Input: part model. Units: mm. Frame: model coordinates. Face numbers are marked on the shaded views. A direction names the side the tool comes from. Give positions to 0.01 mm unless a question says otherwise; leave off trailing zeros. Loops run counter-clockwise (first coordinate to the right, second up) from the corner with the lowest first, then second, coordinate; pieces in that order, holes last. Notation, with made-up numbers: (-18, 72) -> (-6, 72) arc R18 cw to (-6, 90) -> close; hole circle Ø10 at (38, 1). An arc over 180 degrees is marked (long way). Answer as a JSON object with one key per item and string values. Group by question number.
Autodesk Inventor part; units mm, degrees
ref_plane "YZ Plane" through (0, 0, 0) normal (1, 0, 0) x (0, 1, 0)
ref_plane "XZ Plane" through (0, 0, 0) normal (0, 1, 0) x (-1, 0, 0)
ref_plane "XY Plane" through (0, 0, 0) normal (0, 0, 1) x (1, 0, 0)
sketch "Sketch1" plane through (0, 0, 0) normal (0, 0, 1) x (1, 0, 0)
  line L0 (0, 10) -> (0, -10) construction
  line L1 (-4, 10) -> (-4, -10)
  line L2 (4, -10) -> (4, 10)
  arc A0 (4, 10) -> (-4, 10) centre (0, 10) ccw
  arc A1 (-4, -10) -> (4, -10) centre (0, -10) ccw
  circle A2 centre (0, -10) radius 1.5
  line L3 (0, 0) -> (0, 10) construction
  line L4 (1.5, 0) -> (1.5, 10)
  line L5 (-1.5, 10) -> (-1.5, 0)
  arc A3 (-1.5, 0) -> (1.5, 0) centre (0, 0) ccw
  arc A4 (1.5, 10) -> (-1.5, 10) centre (0, 10) ccw
  point P0 (0, 0)
  point P1 (0, 5)
  dimension "d0" = 10
  dimension "d1" = 8
  dimension "d2" = 3
  dimension "d3" = 5
  dimension "d4" = 3
  dimension "d5" = 5
extrude "Extrusion1" add sketch "Sketch1" along normal blind 3.5
properties part number "3DP_PLA_Part_Detector_Mounting_Bracket_Short" material "ABS Plastic"
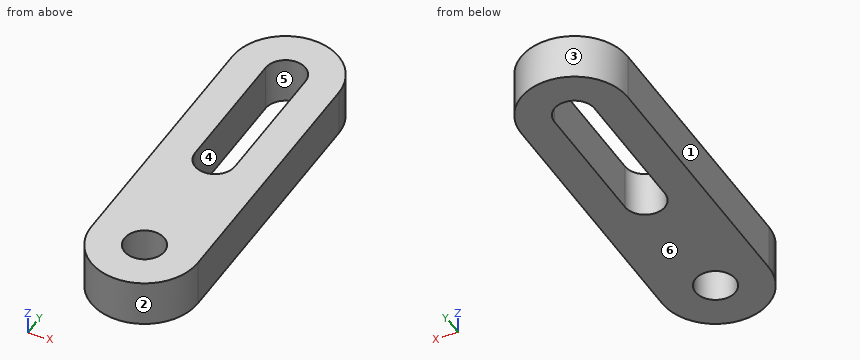
Q1. Section A-A on y = 9.75. Return the cut outline in (x, z), then the cut area to 3 significant figures.
Q2. Section C-C on x = 1. Return the cut outline in (y, z), then the cut area to 3 significant figures.
Q3. Ray query, probe 1 along Y at (x, z) = (0, 0.9); probe 2 along X at (y, z) = (5.25, 3.2); probe 3 along X at (y, z) = (-9, 1.1). Return the intervals inside material, ascending.
Q4. Section D-D on x = 3. Return the cut outline in (y, z), then the cut area to 3 significant figures.
Q5. Pin query (flat end, axial travel): pin 1 Ø1.5 at (x, y) = (-0.5, 6) entering from -Z. Return the tip coordinate at first contact, or that it passes through.
Q6. Pull-direction query (Y, two-part tool) for the marked faces 1, 2, 3 and 4; classes: +Y half, -Y half, draft (parallel to the pull), parting line (faces both ways), or undercut.
Q7. Section B-B on z = 1.9. Return the cut outline in (x, y), then the cut area to 3 significant figures.
Q8. Set-up query: the marked faces 5 and 6. Return all of +Z, -Z, +X, -X, +Y, -Y with unobstructed straight access to the full face (end or side cutting, diameter ignored); none if empty.
Numbers:
{
 "1": {"outline": "(-4, 0) -> (-1.5, 0) -> (-1.5, 3.5) -> (-4, 3.5) -> close; (1.5, 0) -> (4, 0) -> (4, 3.5) -> (1.5, 3.5) -> close", "area": "17.5 mm²"},
 "2": {"outline": "(-13.87, 0) -> (-11.12, 0) -> (-11.12, 3.5) -> (-13.87, 3.5) -> close; (-8.88, 0) -> (-1.12, 0) -> (-1.12, 3.5) -> (-8.88, 3.5) -> close; (11.12, 0) -> (13.87, 0) -> (13.87, 3.5) -> (11.12, 3.5) -> close", "area": "46.5 mm²"},
 "3": {"probe 1": "y = -14 to -11.5, -8.5 to -1.5, 11.5 to 14", "probe 2": "x = -4 to -1.5, 1.5 to 4", "probe 3": "x = -4 to -1.12, 1.12 to 4"},
 "4": {"outline": "(-12.65, 0) -> (12.65, 0) -> (12.65, 3.5) -> (-12.65, 3.5) -> close", "area": "88.5 mm²"},
 "5": {"pin 1": "passes through"},
 "6": {"face 1": "draft", "face 2": "-Y half", "face 3": "+Y half", "face 4": "undercut"},
 "7": {"outline": "(-4, -10) arc R4 ccw to (4, -10) -> (4, 10) arc R4 ccw to (-4, 10) -> close; hole circle Ø3 at (0, -10); hole (-1.5, 0) arc R1.5 ccw to (1.5, 0) -> (1.5, 10) arc R1.5 ccw to (-1.5, 10) -> close", "area": "166 mm²"},
 "8": {"face 5": "+Z, -Z", "face 6": "-Z, +X, -X, +Y, -Y"}
}
